```python
from build123d import *

# Parameters (mm, degrees)
SKETCH_1_R               = 4.5
SKETCH_1_R_2             = 1.5
EXTRUDE_1_DEPTH          = 3
EXTRUDE_1_DEPTH_BACK     = 3
SKETCH_1_R_3             = 4
SKETCH_1_R_4             = 2.5
EXTRUDE_1_2_DEPTH        = 3
EXTRUDE_1_2_DEPTH_BACK   = 3
EXTRUDE_2_REACH          = 26.5
SKETCH_2_R               = 3
SKETCH_3_R               = 3
CUT_EXTRUDE_1_DEPTH      = 10
SKETCH_4_R               = 2
EXTRUDE_3_DEPTH          = 20
CUT_EXTRUDE_2_DEPTH      = 20
CUT_EXTRUDE_2_DEPTH_BACK = 20
SKETCH_7_R               = 2
CUT_EXTRUDE_3_DEPTH      = 30


with BuildPart() as part:
    # Sketch 1 → Extrude 1 (new body, two sides)
    with BuildSketch(Plane(origin=(0, 0, 0), x_dir=(0, 0, -1), z_dir=(1, 0, 0))) as extrude_1_sk:
        with Locations((0, 20)):
            Circle(SKETCH_1_R)
        with Locations((0, 20)):
            Circle(SKETCH_1_R_2, mode=Mode.SUBTRACT)
    extrude(amount=EXTRUDE_1_DEPTH)
    extrude(extrude_1_sk.sketch, amount=-EXTRUDE_1_DEPTH_BACK)

    # Sketch 2 → Extrude 2 (add, up to next)
    with BuildSketch(Plane(origin=(0, 0, 0), x_dir=(1, 0, 0), z_dir=(0, 1, 0)), mode=Mode.PRIVATE) as extrude_2_sk1:
        Circle(SKETCH_2_R)
    extrude_2_tool1 = extrude(extrude_2_sk1.sketch, amount=EXTRUDE_2_REACH, mode=Mode.PRIVATE) - part.part
    add(extrude_2_tool1.solids().sort_by_distance((0, 0, 0))[0])

    # Sketch 3 → Cut-Extrude 1 (cut)
    with BuildSketch(Plane.XZ):
        Circle(SKETCH_3_R)
    extrude(amount=-CUT_EXTRUDE_1_DEPTH, mode=Mode.SUBTRACT)

    # Sketch 4 → Extrude 3 (add)
    with BuildSketch(Plane.XZ.offset(-10)):
        Circle(SKETCH_4_R)
    extrude(amount=EXTRUDE_3_DEPTH)



with BuildPart() as body_2:
    # Sketch 1 → Extrude 1 2 (new body, two sides)
    with BuildSketch(Plane(origin=(0, 0, 0), x_dir=(0, 0, -1), z_dir=(1, 0, 0))) as extrude_1_2_sk:
        with Locations((0, -65)):
            Circle(SKETCH_1_R_3)
        with Locations((0, -65)):
            Circle(SKETCH_1_R_4, mode=Mode.SUBTRACT)
    extrude(amount=EXTRUDE_1_2_DEPTH)
    extrude(extrude_1_2_sk.sketch, amount=-EXTRUDE_1_2_DEPTH_BACK)


with BuildPart() as part_1:
    add(part.part)

    add(body_2.part)  # Revolve 2 merges body 2
    # Sketch 5 → Revolve 2 (revolve)
    with BuildSketch(Plane(origin=(0, 0, 0), x_dir=(0, 0, -1), z_dir=(1, 0, 0))):
        Polygon((0, -10), (4, -10), (6, -17.535898385), (6, -42.535898385), (8.5, -42.535898385), (8.5, -50.535898385), (7, -50.535898385), (7, -56.535898385), (2, -56.535898385), (2, -61.535898385), (0, -61), align=None)
    revolve(axis=Axis((0, -10, 0), (0, -1, 0)))

    # Sketch 6 → Cut-Extrude 2 (cut, two sides)
    with BuildSketch(Plane(origin=(0, 0, 0), x_dir=(0, 0, -1), z_dir=(1, 0, 0))) as cut_extrude_2_sk:
        Polygon((4, -10), (-4, -10), (-9.632301138, 30.288957802), (12.266588859, 30.288957802), align=None)
    extrude(amount=CUT_EXTRUDE_2_DEPTH, mode=Mode.SUBTRACT)
    extrude(cut_extrude_2_sk.sketch, amount=-CUT_EXTRUDE_2_DEPTH_BACK, mode=Mode.SUBTRACT)

    # Sketch 7 → Cut-Extrude 3 (cut)
    with BuildSketch(Plane(origin=(0, -10, 0), x_dir=(1, 0, 0), z_dir=(0, 1, 0))):
        Circle(SKETCH_7_R)
    extrude(amount=-CUT_EXTRUDE_3_DEPTH, mode=Mode.SUBTRACT)


solid = part_1.part
```
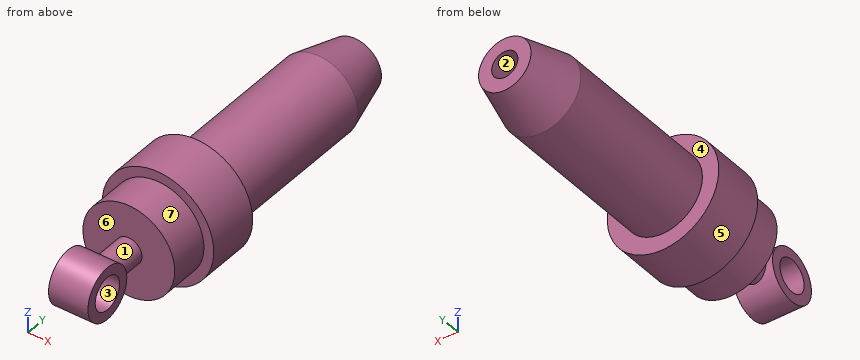
Input: part model. Units: mm. Frame: model coordinates. Face numbers are marked on the shaded views. A direction names the side the tool comes from. Give positions to 0.01 mm unless a question says otherwise; leave off trailing zeros. Loops run counter-clockwise (first coordinate to the right, second up) from the corner with the lowest first, then second, coordinate; pieces in that order, holes last. Notation, with made-up numbers: (33.5, 33.5) -> (78.5, 33.5) arc R17 ccw to (78.5, 66.5) -> close; hole circle Ø3 at (72, 55). An arc over 180 degrees is marked (long way). Use a Markdown table: item, result.
Q1. Section query C-C, the plane y = -65. Return the cut outline in (x, z).
Entries:
| item | result |
|---|---|
| outline | (-3, -4) -> (3, -4) -> (3, -2.5) -> (-3, -2.5) -> close; (-3, 2.5) -> (3, 2.5) -> (3, 4) -> (-3, 4) -> close |
Q2. First-contact query: P1, Ø3.5, axis at x = 0, z = 0, coming from the +Y side; P2, Ø9, axis at y = -65, z = 0, coming from the +X side; P3, Ø6, axis at y = -32, z = -6.5, coming from the -X side; P4, Ø4.5, axis at y = -65, z = 0, coming from the +X side. Flat tips, straight axial feed; report the tip coordinate or a pass-through.
Entries:
| item | result |
|---|---|
| P1 | stops at y = -40 |
| P2 | stops at x = 3 |
| P3 | stops at x = -4.87 |
| P4 | passes through |
Q3. Access query for the marked faces 4, 5, 6 and 7. Directions: +Z, -Z, +X, -X, +Y, -Y. A direction counts if a zero-diameter tool reaches every point of the face in a straight line with its end or side. Return the directions, or none.
Entries:
| item | result |
|---|---|
| face 4 | +Y |
| face 5 | +Y, -Y |
| face 6 | none |
| face 7 | -Y |
Q4. Section query B-B, the plane x = 0. Return the cut outline in (y, z), plus the area to 3 significant figures.
Entries:
| item | result |
|---|---|
| outline | (-61.54, -2) -> (-56.54, -2) -> (-56.54, -7) -> (-50.54, -7) -> (-50.54, -8.5) -> (-42.54, -8.5) -> (-42.54, -6) -> (-17.54, -6) -> (-10, -4) -> (-10, -2) -> (-40, -2) -> (-40, 2) -> (-10, 2) -> (-10, 4) -> (-17.54, 6) -> (-42.54, 6) -> (-42.54, 8.5) -> (-50.54, 8.5) -> (-50.54, 7) -> (-56.54, 7) -> (-56.54, 2) -> (-61.54, 2) arc R4 ccw (long way) to start; hole circle Ø5 at (-65, 0) |
| area | 525 mm² |
Q5. Ray query, probe 1 along X at (y, z) = (-32.5, 0); probe 2 along X at (y, z) = (-56, 5.75); probe 3 along Y at (x, z) = (0, -0.25). Return the intervals inside material, ascending. Write a range as from..to.
Entries:
| item | result |
|---|---|
| probe 1 | x = -6..-2, 2..6 |
| probe 2 | x = -3.99..3.99 |
| probe 3 | y = -68.99..-67.49, -62.51..-40 |
Q6. Section query D-D, the plane y = -37. Return the cut outline in (x, z), plus the area to 3 significant figures.
Entries:
| item | result |
|---|---|
| outline | circle Ø12 at (0, 0); hole circle Ø4 at (0, 0) |
| area | 101 mm² |
Q7. Pull-direction query (X, two-part tool) for the marked faces 1, 2 and 3; classes: pulls with the +X half, pulls with the -X half, needs draft (parallel to the pull), parting line crosses it, or undercut.
Entries:
| item | result |
|---|---|
| face 1 | parting line crosses it |
| face 2 | undercut |
| face 3 | needs draft |
